```python
from build123d import *

# Parameters (mm, degrees)
SKETCH_W  = 400
SKETCH_H  = 200
SKETCH_R  = 1.5625
PAD_DEPTH = 12
FILLET_R  = 3


with BuildPart() as part:
    # Sketch → Pad (new body)
    with BuildSketch(Plane.XY):
        with Locations((200, 100)):
            Rectangle(SKETCH_W, SKETCH_H)
        with Locations((85, 15)):
            Circle(SKETCH_R, mode=Mode.SUBTRACT)
        with Locations((105, 15)):
            Circle(SKETCH_R, mode=Mode.SUBTRACT)
        with Locations((75, 25)):
            Circle(SKETCH_R, mode=Mode.SUBTRACT)
        with Locations((95, 25)):
            Circle(SKETCH_R, mode=Mode.SUBTRACT)
        with Locations((155, 15)):
            Circle(SKETCH_R, mode=Mode.SUBTRACT)
        with Locations((135, 15)):
            Circle(SKETCH_R, mode=Mode.SUBTRACT)
        with Locations((145, 25)):
            Circle(SKETCH_R, mode=Mode.SUBTRACT)
        with Locations((165, 25)):
            Circle(SKETCH_R, mode=Mode.SUBTRACT)
        with Locations((85, 185)):
            Circle(SKETCH_R, mode=Mode.SUBTRACT)
        with Locations((105, 185)):
            Circle(SKETCH_R, mode=Mode.SUBTRACT)
        with Locations((75, 175)):
            Circle(SKETCH_R, mode=Mode.SUBTRACT)
        with Locations((95, 175)):
            Circle(SKETCH_R, mode=Mode.SUBTRACT)
        with Locations((155, 185)):
            Circle(SKETCH_R, mode=Mode.SUBTRACT)
        with Locations((135, 185)):
            Circle(SKETCH_R, mode=Mode.SUBTRACT)
        with Locations((145, 175)):
            Circle(SKETCH_R, mode=Mode.SUBTRACT)
        with Locations((165, 175)):
            Circle(SKETCH_R, mode=Mode.SUBTRACT)
        with BuildLine():
            Line((17.211533, 123.076019), (32.421267, 123.076019))
            ThreePointArc((38.702517, 97.693395), (44.851125, 112.683445), (32.421267, 123.076019))
            ThreePointArc((35.228252, 66.093052), (49.45239, 80.520354), (38.702517, 97.693395))
            Line((35.228252, 66.093052), (17.211533, 66.093052))
            Line((17.211533, 66.093052), (17.211533, 123.076019))
        make_face(mode=Mode.SUBTRACT)
        with BuildLine():
            Line((66.260755, 65.953049), (54.781403, 65.953049))
            Line((54.781403, 65.953049), (54.781403, 122.551093))
            Line((74.352173, 122.551093), (54.781403, 122.551093))
            ThreePointArc((74.351683, 92.765599), (89.613073, 107.658094), (74.352173, 122.551093))
            Line((94.033974, 66.33828), (74.351683, 92.765599))
            Line((83.779968, 66.33828), (94.033974, 66.33828))
            Line((66.260755, 89.596498), (83.779968, 66.33828))
            Line((66.260755, 89.596498), (66.260755, 65.953049))
        make_face(mode=Mode.SUBTRACT)
    extrude(amount=PAD_DEPTH)

    # Fillet
    fillet_edges = [part.edges().sort_by_distance(p)[0] for p in [
        (0, 0, 6),
        (400, 0, 6),
        (400, 200, 6),
        (0, 200, 6),
    ]]
    fillet(fillet_edges, radius=FILLET_R)


solid = part.part
```
Model file for the job. Use its own axes, mm. A direction names the side the tool comes from. Round coordinates to 2 decimals unless told otherwise and drop trailing zeros. Use CSV: the item, a comma, the result in double quotes.
Item 1: Pull direction Y, two halves, no side cores. Call faces 1 (the face through (89, 66.338, 6)), 2 (the face through (197, 101, 0)), 3 (the face through (197, 200, 6)): released by +Y, released by -Y, zero draft, split by the parting line, or undercut.
Worked answers:
face 1,"undercut"
face 2,"zero draft"
face 3,"released by +Y"
Item 2: Saw through at A-A (z = 6.5). State how many separate pieces and enclosed holes the cut face has, plus the area to 3 significant figures.
Worked answers:
separate pieces,"1"
enclosed holes,"18"
area,"76,800 mm²"
Item 3: Probe probe 1 along Y at (x, z) = (165, 4.5); probe 2 along X at (y, z) = (175, 4); probe 3 along Y at (x, z) = (155, 6). List the from-to ranges inside material, lowest first.
Worked answers:
probe 1,"0 to 23.44, 26.56 to 173.44, 176.56 to 200"
probe 2,"0 to 73.44, 76.56 to 93.44, 96.56 to 143.44, 146.56 to 163.44, 166.56 to 400"
probe 3,"0 to 13.44, 16.56 to 183.44, 186.56 to 200"
Item 4: Which spindle directions (+Z, -Z, +X, -X, +Y, -Y) get a long thin tool onto all of the face, cutting with end or side? Do faces 4 (the face through (84.33, 79.37, 5.92)), 5 (the face through (197, 101, 12)). Say none if no direction does.
Worked answers:
face 4,"+Z, -Z"
face 5,"+Z, +X, -X, +Y, -Y"
Item 5: Pin check, flat tip, straight feed: pin 1 (3.5 mm diameter, centred on x = 105, y = 15, fed in from -Z). Stop position of the tip, or through.
Worked answers:
pin 1,"z = 0"
